from build123d import *

# Parameters (mm, degrees)
IZIM2_R                     = 82.5
IZIM2_R_2                   = 27
Y_KSEKLIK_EKSTR_ZYON1_DEPTH = 20
IZIM3_R                     = 8
KES_EKSTR_ZYON1_DEPTH       = 20
IZIM4_R                     = 43
IZIM4_R_2                   = 27


with BuildPart() as part:
    # Çizim2 → Yükseklik-Ekstrüzyon1 (new body)
    with BuildSketch(Plane.XY):
        Circle(IZIM2_R)
        Circle(IZIM2_R_2, mode=Mode.SUBTRACT)
    y_kseklik_ekstr_zyon1 = extrude(amount=Y_KSEKLIK_EKSTR_ZYON1_DEPTH)

    # Çizim3 → Kes-Ekstrüzyon1 (cut)
    with BuildSketch(Plane.XY.offset(20)):
        with Locations((0, 63)):
            Circle(IZIM3_R)
        with Locations((44.547727215, 44.547727215)):
            Circle(IZIM3_R)
        with Locations((63, 0)):
            Circle(IZIM3_R)
        with Locations((44.547727215, -44.547727215)):
            Circle(IZIM3_R)
        with Locations((0, -63)):
            Circle(IZIM3_R)
        with Locations((-44.547727215, -44.547727215)):
            Circle(IZIM3_R)
        with Locations((-63, 0)):
            Circle(IZIM3_R)
        with Locations((-44.547727215, 44.547727215)):
            Circle(IZIM3_R)
    kes_ekstr_zyon1 = extrude(amount=-KES_EKSTR_ZYON1_DEPTH, mode=Mode.SUBTRACT)

    # Süpür1: sweep along a path in Çizim5
    with BuildLine(Plane(origin=(0, 0, 0), x_dir=(0, 0, -1), z_dir=(1, 0, 0))) as s_p_r1_path:
        ThreePointArc((0, 0), (63.639610307, 26.360389693), (90, 90))
    # Çizim4 → Süpür1 (sweep)
    with BuildSketch(Plane(origin=(0, 0, 0), x_dir=(-1, 0, 0), z_dir=(0, 0, -1))):
        Circle(IZIM4_R)
        Circle(IZIM4_R_2, mode=Mode.SUBTRACT)
    sweep(path=s_p_r1_path.line)

    # Aynalama3: Yükseklik-Ekstrüzyon1, Kes-Ekstrüzyon1 across plane
    add(y_kseklik_ekstr_zyon1.mirror(Plane(origin=(0, 45, -45), x_dir=(0, 0.7071067811865475, 0.7071067811865477), z_dir=(0, -0.7071067811865476, 0.7071067811865475))))
    add(kes_ekstr_zyon1.mirror(Plane(origin=(0, 45, -45), x_dir=(0, 0.7071067811865475, 0.7071067811865477), z_dir=(0, -0.7071067811865476, 0.7071067811865475))), mode=Mode.SUBTRACT)


solid = part.part
Verification items for the finished model (mm, model axes). A direction names the side the tool comes from. Coordinates: 2 decimals unless noted, no trailing zeros. Write each loop counter-clockwise with the first axis right and the second up, starting at its lowest first coordinate (ties: lowest second). Pieces come first, ordered by that corner, then holes. Notation, with made-up numbers: (58, -7.75) - (74, -7.75) arc R31 ccw to (74, 25.25) - close; hole circle Ø1 at (-38, 54). An arc over 180 degrees is marked (long way). Answer as a JSON object with one key per item and string values.
(1) Gauge pin test, flat ends, axial feed: pin 1 Ø14.5 at (x, z) = (-44.55, -134.55) entering from -Y; pin 2 Ø10 at (x, y) = (9, -15) entering from -Z; pin 3 Ø14.5 at (x, y) = (0, 63) entering from -Z; pin 4 Ø21 at (x, y) = (44.55, -44.55) entering from -Z. Record the tip position at first contact, or that the pin passes through.
Report:
{"pin 1": "through", "pin 2": "z = -86.43", "pin 3": "z = -131.53", "pin 4": "z = 0"}
(2) Mould release check, pull along X, two halves, no side actions. Record for faces 1 (the cylindrical face through (-1.041, 70.932, 10.14)), 2 (the flat face through (-19.5, 19.5, 20)), 3 (the cylindrical face through (-10.74, 99.86, -8.202)): pulls with the +X half, pulls with the -X half, needs draft (parallel to the pull), parting line crosses it, or undercut.
Report:
{"face 1": "undercut", "face 2": "needs draft", "face 3": "parting line crosses it"}
(3) Cross-section at A-A on x = 14.5. Record the cut outline in (y, z), plus the area to 3 significant figures.
Report:
{"outline": "(-81.22, 0) - (-40.48, 0) arc R130.48 ccw to (90, -130.48) - (90, -171.22) - (110, -171.22) - (110, -112.78) - (90, -112.78) arc R112.78 cw to (-22.78, 0) - (-22.78, 20) - (-81.22, 20) - close; (22.78, 0) arc R67.22 ccw to (90, -67.22) - (110, -67.22) - (110, -8.78) - (90, -8.78) - (90, -49.52) arc R49.52 cw to (40.48, 0) - (81.22, 0) - (81.22, 20) - (22.78, 20) - close", "area": "9,680 mm^2"}
(4) Thickness scan on line 1 along Z through (x, y) = (0, 99); line 2 along Y through (x, z) = (0, 4); line 3 along X through (y, z) = (45.5, -77.5). Record the ranges inside material, lowest first.
Report:
{"line 1": "-172.5 to -161, -145 to -117, -63 to -35, -19 to -7.5", "line 2": "-82.5 to -71, -55 to -27, 27 to 55, 71 to 82.5", "line 3": "-43 to -26.99, 26.99 to 43"}
(5) Cross-section at B-B on y = -63. Record the cut outline in (x, z).
Report:
{"outline": "(-53.27, 0) - (-8, 0) - (-8, 20) - (-53.27, 20) - close; (8, 0) - (53.27, 0) - (53.27, 20) - (8, 20) - close"}
(6) Cross-section at C-C on z = -90. Give the number of separate pieces and of enclosed holes in the cut face, plus the area to 3 significant figures.
Report:
{"separate pieces": "3", "enclosed holes": "0", "area": "5,320 mm^2"}
(7) Cross-section at D-D on x = 67.5. Record the cut outline in (y, z), plus the area to 3 significant figures.
Report:
{"outline": "(-47.43, 0) - (-6.61, 0) - (-6.61, 20) - (-47.43, 20) - close; (6.61, 0) - (47.43, 0) - (47.43, 20) - (6.61, 20) - close; (90, -137.43) - (110, -137.43) - (110, -96.61) - (90, -96.61) - close; (90, -83.39) - (110, -83.39) - (110, -42.57) - (90, -42.57) - close", "area": "3,270 mm^2"}
(8) Tool access check on faces 4 (the cylindrical face through (-40.856, -51.645, 10.14)), 5 (the flat face through (36, 90, -126)), 6 (the cylindrical face through (7.63, 100.14, -24.6)), 7 (the cylindrical face through (-40.247, 51.293, 10.14)). Record the directions out of +Z, -Z, +X, -X, +Y, -Y that give a thin tool (end or side, any length) a straight path to the whole face; none if there is none.
Report:
{"face 4": "+Z, -Z", "face 5": "none", "face 6": "+Y", "face 7": "+Z"}
